Study the drawing (mm; zero at the part's minimum x, y, z) and answer. A direction names the side the tool comes from. Round coordinates to 2 decimals unless told otherwise and drop trailing zeros. Write each loop counter-clockwise with the first axis right and the second up, starting at its lowest first coordinate (ties: lowest second). Pieces come first, ordered by that corner, then holes. Notation, with made-up numbers: M 42,-16 L 51,-16 A8 cw 51,-12 Z; hole C 13.5,-19 d11. An arc over 180 degrees is marked long. Put each result on its own line as item: value. Start each with the question number.
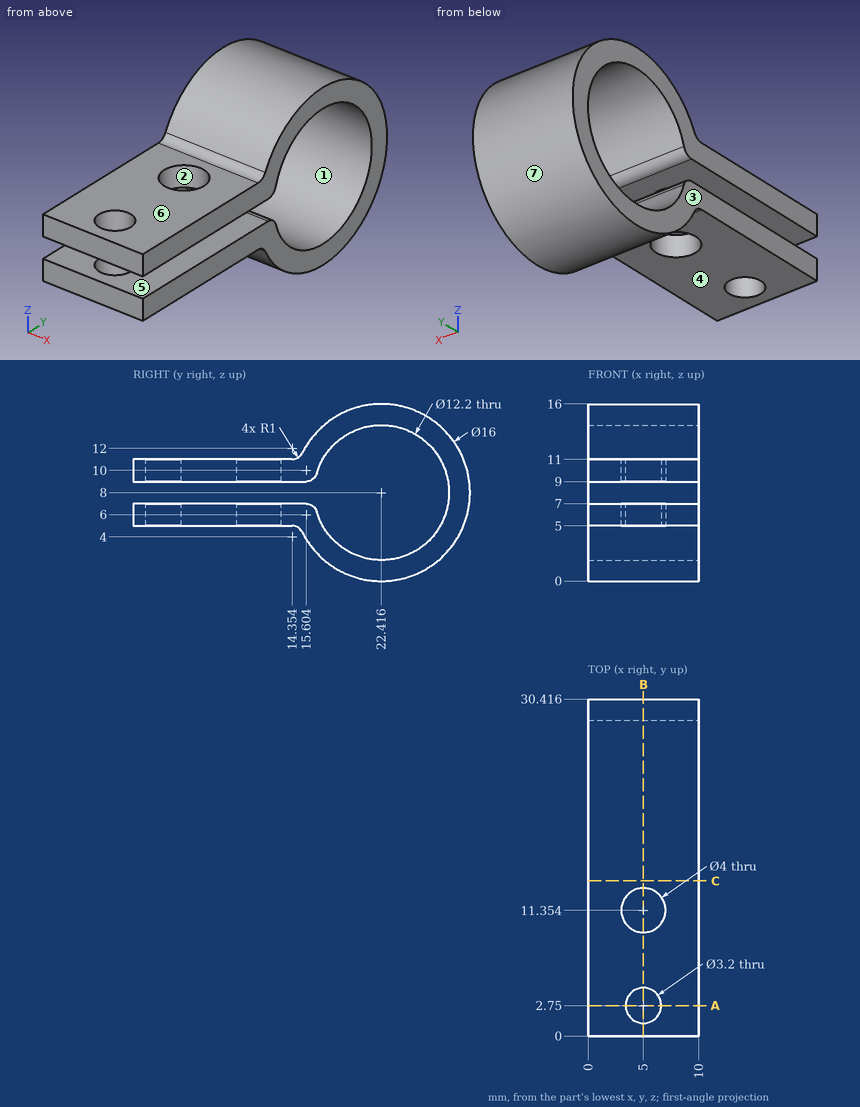
Item 1: Section B-B (x = 5) is taken. Count the separate pieces of the cut face and the enclosed holes in it, and give its area (3 significant figures).
Item 2: Which of the six approach directions +Z, -Z, +X, -X, +Y, -Y give full straight-line access (tool end or side, diameter ignored) to the marked faces 4, 5, 6 and 7?
Item 3: Section C-C (y = 14) is taken. Give the vertices of the cut face in (x, z).
Item 4: Determine the mould class of the marked faces 1, 2 and 3 for opening direction X: released by +X, released by -X, zero draft, split by the parting line, or undercut.
Item 5: Section A-A (y = 2.75) is taken. Give the vertices of the cut face in (x, z), and give its area (3 significant figures).
Item 6: Consider line 1 along Y through (x, z) = (5, 10); line 2 along Z through (x, y) = (6.5, 4.5); line 3 along Z through (x, y) = (1.5, 24). Determine where each line is inside the solid, lowest interval first. Write a range as [from, to].
Item 7: Flat-ended cylindrical pins translate along their axes: pin 1 (1 mm diameter, centred on x = 5, y = 15, fed in from +Z); pin 2 (3 mm diameter, centred on x = 2.5, y = 10.5, fed in from +Z); pin 3 (3.5 mm diameter, centred on x = 5, y = 2.75, fed in from -Z). Find the tip coordinate at first contact, or state that the pin passes through.
Output values:
1. separate pieces: 5
1. enclosed holes: 0
1. area: 110 mm^2
2. face 4: -Z, +X, -X, -Y
2. face 5: +X, -X, -Y
2. face 6: +Z, +X, -X, -Y
2. face 7: +X, -X
3. outline: M 0,5 L 10,5 L 10,7 L 0,7 Z; M 0,9 L 10,9 L 10,11 L 0,11 Z
4. face 1: zero draft
4. face 2: undercut
4. face 3: released by -X
5. outline: M 0,5 L 3.4,5 L 3.4,7 L 0,7 Z; M 0,9 L 3.4,9 L 3.4,11 L 0,11 Z; M 6.6,5 L 10,5 L 10,7 L 6.6,7 Z; M 6.6,9 L 10,9 L 10,11 L 6.6,11 Z
5. area: 27.2 mm^2
6. line 1: y = [0, 1.15], [4.35, 9.35], [13.35, 16.65], [28.18, 30.16]
6. line 2: z = [5, 7], [9, 11]
6. line 3: z = [0.16, 2.11], [13.89, 15.84]
7. pin 1: stops at z = 12.02
7. pin 2: stops at z = 11
7. pin 3: stops at z = 5
